from build123d import *

# Parameters (mm, degrees)
EXTRUDE1_DEPTH = 76.2


with BuildPart() as part:
    # Sketch1 → Extrude1 (new body)
    with BuildSketch(Plane(origin=(0, 0, 0), x_dir=(0, 0, -1), z_dir=(1, 0, 0))):
        Polygon((0, 0), (66.893951326, 0), (66.893951326, 55.885931794), (59.273951326, 55.885931794), (59.273951326, 7.62), (0, 7.62), align=None)
    extrude(amount=-EXTRUDE1_DEPTH)


solid = part.part
Geometry check sheet. Reference: the model listing, model coordinates, mm. A direction names the side the tool comes from. Round coordinates to 2 decimals unless told otherwise and drop trailing zeros. Loops run counter-clockwise (first coordinate to the right, second up) from the corner with the lowest first, then second, coordinate; pieces in that order, holes last. Notation, with made-up numbers: (55, 49.5) - (87, 49.5) arc R20 cw to (87, 68.5) - close; hole circle Ø1 at (-38.5, 61). An arc over 180 degrees is marked (long way). Answer as CSV lines item,"result".
(1) Cross-section at A-A, the plane y = 47. Enter the section's corners in (x, z), and give its area (3 significant figures).
Output values:
outline,"(-76.2, -66.89) - (0, -66.89) - (0, -59.27) - (-76.2, -59.27) - close"
area,"581 mm²"
(2) Depth check by flat-ended pin: pin 1 Ø18 at (x, z) = (-19, -36.5) entering from +Y. Enter the tip coordinate at first touch or a pass-through.
Output values:
pin 1,"stops at y = 7.62"
(3) Cross-section at C-C, the plane z = -51.5. Enter the section's corners in (x, y).
Output values:
outline,"(-76.2, 0) - (0, 0) - (0, 7.62) - (-76.2, 7.62) - close"
(4) Material ranges on line 1 along Z through (x, y) = (-69.5, 14.5); line 2 along Y through (x, z) = (-14, -50.5), recorded low to high.
Output values:
line 1,"z = -66.89 to -59.27"
line 2,"y = 0 to 7.62"
(5) Cross-section at B-B, the plane x = -33.5. Enter the section's corners in (y, z), and give its area (3 significant figures).
Output values:
outline,"(0, -66.89) - (55.89, -66.89) - (55.89, -59.27) - (7.62, -59.27) - (7.62, 0) - (0, 0) - close"
area,"878 mm²"
(6) Set-up check for faces 1 (the face through (-38, 28, -66.894)), 2 (the face through (-38, 32, -59.274)): record each of +Z, -Z, +X, -X, +Y, -Y from which the full face is reachable in a straight line by a thin tool's end or side.
Output values:
face 1,"-Z, +X, -X, +Y, -Y"
face 2,"+Z, +X, -X, +Y"
